```python
from build123d import *

# Parameters (mm, degrees)
SKETCH_1_W                   = 100
SKETCH_1_H                   = 90.5
EXTRUDE_1_DEPTH              = 50
SKETCH_2_W                   = 15
SKETCH_2_H                   = 70.5
CUT_EXTRUDE_1_DEPTH          = 144.841058116
SKETCH_4_R                   = 4.85
CUT_EXTRUDE_3_DEPTH          = 144.841058116
HOLE_WIZARD_M6_1_D           = 7
HOLE_WIZARD_M6_1_CBORE_D     = 11
HOLE_WIZARD_M6_1_CBORE_DEPTH = 6
HOLE_WIZARD_M3_1_D           = 2.5
HOLE_WIZARD_M3_1_DEPTH       = 7.5
HOLE_WIZARD_M3_1_TIP         = 0.751075774


with BuildPart() as part:
    # 草图1 → 凸台-拉伸1 (new body)
    with BuildSketch(Plane.XY):
        with Locations((50, 45.25)):
            Rectangle(SKETCH_1_W, SKETCH_1_H)
    extrude(amount=EXTRUDE_1_DEPTH)

    # 草图2 → 切除-拉伸1 (cut, through all)
    with BuildSketch(Plane.ZY):
        with Locations((7.5, 35.25)):
            Rectangle(SKETCH_2_W, SKETCH_2_H)
    extrude(amount=-CUT_EXTRUDE_1_DEPTH, mode=Mode.SUBTRACT)

    # 草图4 → 切除-拉伸3 (cut, through all)
    with BuildSketch(Plane(origin=(0, 90.5, 0), x_dir=(1, 0, 0), z_dir=(0, 1, 0))):
        with Locations((15, -3)):
            Circle(SKETCH_4_R)
        with Locations((55, -3)):
            Circle(SKETCH_4_R)
    extrude(amount=-CUT_EXTRUDE_3_DEPTH, mode=Mode.SUBTRACT)

    # M6 六角凹头螺钉的柱形沉头孔1 (through all)
    with Locations(Plane(origin=(0, 90.5, 0), x_dir=(-1, 0, 0), z_dir=(0, 1, 0))):
        with Locations((-30, 35), (-70, 35)):
            CounterBoreHole(HOLE_WIZARD_M6_1_D / 2, HOLE_WIZARD_M6_1_CBORE_D / 2, HOLE_WIZARD_M6_1_CBORE_DEPTH)

    # M3 螺纹孔1
    with Locations(Plane.ZY):
        with Locations((39, 65.5), (19.5, 65.5)):
            Hole(HOLE_WIZARD_M3_1_D / 2, depth=HOLE_WIZARD_M3_1_DEPTH)
            with Locations((0, 0, -(HOLE_WIZARD_M3_1_DEPTH + HOLE_WIZARD_M3_1_TIP / 2))):  # 118° drill point
                Cone(0, HOLE_WIZARD_M3_1_D / 2, HOLE_WIZARD_M3_1_TIP, mode=Mode.SUBTRACT)


solid = part.part
```
Here's how the part is built. I have some questions about the finished solid (model axes, mm). A direction names the side the tool comes from. Coordinates: 2 decimals unless noted, no trailing zeros. Order: outer loops, then holes, each group sorted by start corner. A loop starts at its lowest first (then second) coordinate and runs counter-clockwise, first axis right, second up.
1) Imagine slicing it at D-D on x = 48.5. List the corners of the cut face in (y, z) for me.
2) We'd pull the mould along X, two halves only. Please class faces 1 (the face through (49, 0, 32)), 2 (the face through (100, 45, 30)), 3 (the face through (14.848, 80.64, 7.848)): +X half, -X half, draft (parallel to the pull), parting line (faces both ways), or undercut.
3) I need wall thicknesses on line 1 (Z direction, x = 30, y = 32); line 2 (X direction, y = 85, z = 36); line 3 (Z direction, x = 30, y = 89). Which ranges of each line are inside material? Lowest first, please.
4) Will these pins go through, and if not, where does the flat tip stop? pin 1 (6 mm diameter, centred on x = 17, z = 5.5, fed in from -Y); pin 2 (8 mm diameter, centred on x = 30, z = 35, fed in from +Y); pin 3 (3 mm diameter, centred on x = 42.5, y = 41, fed in from -Z); pin 4 (8 mm diameter, centred on x = 15, z = 3, fed in from +Y).
5) Imagine slicing it at C-C on y = 39. List the corners of the cut face in (x, z) for me.
6) Imagine slicing it at B-B on x = 70. List the corners of the cut face in (y, z) for me, and give its area (3 significant figures).
7) Imagine slicing it at A-A on z = 35. List the corners of the cut face in (x, y) for me.
8) Which directions (+Z, -Z, +X, -X, +Y, -Y) give clear straight access to the entire face, cutting with the end or side of a thin tool? Please do faces 4 (the face through (75.495, 87.542, 35.242)), 5 (the face through (29.54, 41.66, 38.47)), 6 (the face through (49, 35, 15)), 7 (the face through (3.8, 66.74, 39.16)).
Response values:
1. outline: (0, 15) - (70.5, 15) - (70.5, 0) - (90.5, 0) - (90.5, 50) - (0, 50) - close
2. face 1: draft
2. face 2: +X half
2. face 3: undercut
3. line 1: z = 15 to 31.5, 38.5 to 50
3. line 2: x = 0 to 24.59, 35.41 to 64.59, 75.41 to 100
3. line 3: z = 0 to 29.5, 40.5 to 50
4. pin 1: stops at y = 70.5
4. pin 2: stops at y = 84.5
4. pin 3: stops at z = 15
4. pin 4: passes through
5. outline: (0, 15) - (100, 15) - (100, 50) - (0, 50) - close; hole circle Ø7 at (30, 35); hole circle Ø7 at (70, 35)
6. outline: (0, 15) - (70.5, 15) - (70.5, 0) - (90.5, 0) - (90.5, 29.5) - (84.5, 29.5) - (84.5, 31.5) - (0, 31.5) - close; (0, 38.5) - (84.5, 38.5) - (84.5, 40.5) - (90.5, 40.5) - (90.5, 50) - (0, 50) - close
6. area: 2,810 mm2
7. outline: (0, 0) - (26.5, 0) - (26.5, 84.5) - (24.5, 84.5) - (24.5, 90.5) - (0, 90.5) - close; (33.5, 0) - (66.5, 0) - (66.5, 84.5) - (64.5, 84.5) - (64.5, 90.5) - (35.5, 90.5) - (35.5, 84.5) - (33.5, 84.5) - close; (73.5, 0) - (100, 0) - (100, 90.5) - (75.5, 90.5) - (75.5, 84.5) - (73.5, 84.5) - close
8. face 4: +Y
8. face 5: +Y, -Y
8. face 6: -Z, +X, -X, -Y
8. face 7: -X
